Can you work these out from the model? Positions are in its coordinate system, mm. A direction names the side the tool comes from. Coordinates: 2 decimals unless noted, no trailing zeros. Write each loop counter-clockwise with the first axis right and the second up, starting at its lowest first coordinate (ties: lowest second). Pieces come first, ordered by that corner, then holes. Notation, with made-up numbers: (56.5, 11.5) - (108.5, 11.5) arc R35 cw to (108.5, 45.5) - close; hole circle Ø3 at (83, -38.75). An arc over 180 degrees is marked (long way). One line per question, with ' | ' between items. Start each with the question number.
from build123d import *

# Parameters (mm, degrees)
BOSS_EXTRUDE1_DEPTH             = 711.2
SKETCH3_R                       = 3.175
SASH_ADJUSTMENT_HOLES_CUT_DEPTH = 775.037716398
LPATTERN1_COUNT                 = 6
LPATTERN1_PITCH                 = 101.6
SKETCH4_R                       = 1.5875
MOUNTING_SCREW_HOLES_CUT_DEPTH  = 857.308742511
LPATTERN2_COUNT                 = 7
LPATTERN2_PITCH                 = 101.6


with BuildPart() as part:
    # Sketch2 → Boss-Extrude1 (new body)
    with BuildSketch(Plane(origin=(0, 0, 0), x_dir=(1, 0, 0), z_dir=(0, 1, 0))):
        Polygon((-438.15, -304.8), (-438.15, -292.1), (-458.7875, -292.1), (-458.7875, -285.75), (-438.15, -285.75), (-438.15, -279.4), (-476.25, -279.4), (-476.25, -304.8), align=None)
    extrude(amount=BOSS_EXTRUDE1_DEPTH)

    # Sketch3 → Sash Adjustment Holes Cut (cut, through all)
    with BuildSketch(Plane(origin=(-458.7875, 0, 0), x_dir=(0, 0, -1), z_dir=(1, 0, 0))):
        with Locations((-288.925, 609.6)):
            Circle(SKETCH3_R)
    sash_adjustment_holes_cut = extrude(amount=-SASH_ADJUSTMENT_HOLES_CUT_DEPTH, mode=Mode.SUBTRACT)

    # LPattern1: Sash Adjustment Holes Cut ×6
    with Locations(*[(0, -i * LPATTERN1_PITCH, 0) for i in range(1, LPATTERN1_COUNT)]):
        add(sash_adjustment_holes_cut, mode=Mode.SUBTRACT)

    # Sketch4 → Mounting Screw Holes Cut (cut, through all)
    with BuildSketch(Plane.XY.offset(304.8)):
        with Locations((-467.51875, 50.8)):
            Circle(SKETCH4_R)
    mounting_screw_holes_cut = extrude(amount=-MOUNTING_SCREW_HOLES_CUT_DEPTH, mode=Mode.SUBTRACT)

    # LPattern2: Mounting Screw Holes Cut ×7
    with Locations(*[(0, i * LPATTERN2_PITCH, 0) for i in range(1, LPATTERN2_COUNT)]):
        add(mounting_screw_holes_cut, mode=Mode.SUBTRACT)


solid = part.part
(1) If I drill on probe 1 along Z at (x, y) = (-440.5, 585.5); probe 2 along X at (y, z) = (152.4, 296.5); probe 3 along X at (y, z) = (77, 291.25), over which ranges is the centre line in solid material (lowest first)?
(2) If we section it at A-A on x = -447.5: List the corners of the cut face in (y, z) for me, plus the area to 3 significant figures.
(3) I'm going to push a flat-ended pin straight in: pin 1 (3 mm diameter, centred on y = 681.5, z = 289.5, fed in from +X). Where does the tip first touch, or does it pass through?
(4) If we mould it in two halves opening along Z, with no side actions, what happens to faces 3 (the face through (-476.25, 351, 292)), 4 (the face through (-457, 351, 304.8)), 5 (the face through (-449, 351, 285.75))? For each: +Z half, -Z half, draft (parallel to the pull), parting line (faces both ways), or undercut.
(5) Which directions (+Z, -Z, +X, -X, +Y, -Y) give clear straight access to the entire face, cutting with the end or side of a thin tool? Please do faces 1 (the face through (-448, 351, 292.1)), 2 (the face through (-457, 351, 279.4)).
(6) If we section it at B-B on y = 626: List the corners of the cut face in (x, z) for me, plus the area to 3 significant figures.
Values:
1) probe 1: 279.4 to 285.75, 292.1 to 304.8 | probe 2: -476.25 to -469.11, -465.93 to -438.15 | probe 3: -476.25 to -458.79
2) outline: (0, 279.4) - (711.2, 279.4) - (711.2, 285.75) - (0, 285.75) - close; (0, 292.1) - (711.2, 292.1) - (711.2, 304.8) - (0, 304.8) - close | area: 13,500 mm2
3) pin 1: x = -458.79
4) face 3: draft | face 4: +Z half | face 5: undercut
5) face 1: +X, +Y, -Y | face 2: -Z, +X, -X, +Y, -Y
6) outline: (-476.25, 279.4) - (-438.15, 279.4) - (-438.15, 285.75) - (-458.79, 285.75) - (-458.79, 292.1) - (-438.15, 292.1) - (-438.15, 304.8) - (-476.25, 304.8) - close | area: 837 mm2
